Design review of the part built by this model. Coordinates are the model's own, in mm. Face numbers are marked on the shaded views. A direction names the side the tool comes from. Round coordinates to 2 decimals unless told otherwise and drop trailing zeros. Order: outer loops, then holes, each group sorted by start corner. A loop starts at its lowest first (then second) coordinate and runs counter-clockwise, first axis right, second up. Notation, with made-up numbers: M 39,41.25 L 59,41.25 A25 ccw 59,65.25 Z; hole C 11.5,14.5 d5. An arc over 180 degrees is marked long. Write item = value, one per line. Start each with the question number.
```python
from build123d import *

# Parameters (mm, degrees)
SKETCH_1_W          = 15
SKETCH_1_H          = 50
EXTRUDE_1_DEPTH     = 8
SKETCH_2_R          = 1.5
CUT_EXTRUDE_1_DEPTH = 28.299267389
CUT_EXTRUDE_3_DEPTH = 28.299267389


with BuildPart() as part:
    # 草图1 → 凸台-拉伸1 (new body)
    with BuildSketch(Plane.XY):
        Rectangle(SKETCH_1_W, SKETCH_1_H)
    extrude(amount=EXTRUDE_1_DEPTH)

    # 草图2 → 切除-拉伸1 (cut, through all)
    with BuildSketch(Plane.XY.offset(8)):
        with Locations((-4, 21)):
            Circle(SKETCH_2_R)
        with Locations((4, 21)):
            Circle(SKETCH_2_R)
        with Locations((4, -21)):
            Circle(SKETCH_2_R)
        with Locations((-4, -21)):
            Circle(SKETCH_2_R)
    extrude(amount=-CUT_EXTRUDE_1_DEPTH, mode=Mode.SUBTRACT)

    # 草图3 → 切除-拉伸3 (cut, through all)
    with BuildSketch(Plane.XY.offset(8)):
        with BuildLine():
            Line((3.5, 15), (3.5, -15))
            ThreePointArc((3.5, -15), (0, -18.5), (-3.5, -15))
            Line((-3.5, -15), (-3.5, 15))
            ThreePointArc((-3.5, 15), (0, 18.5), (3.5, 15))
        make_face()
    extrude(amount=-CUT_EXTRUDE_3_DEPTH, mode=Mode.SUBTRACT)


solid = part.part
```
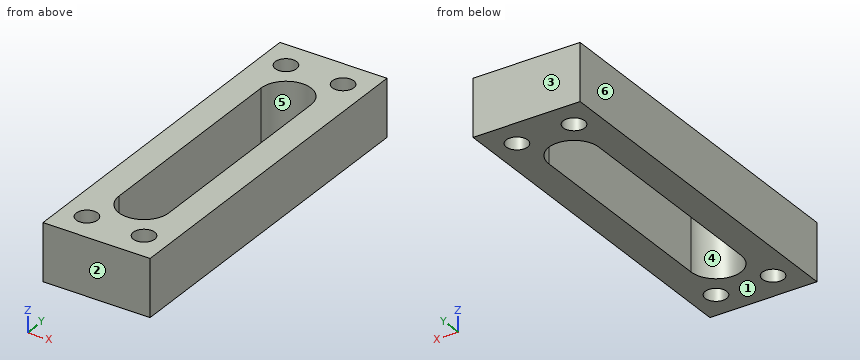
(1) For the marked faces 5 and 6, list the 3-axis set-ups (+Z, -Z, +X, -X, +Y, -Y) from which the entire face can be reached by the end or side of a thin tool; tool diameter is ignored.
(2) Consider section D-D, the plane y = 6. Write out the cut boundary in (x, z), then the cut area to 3 significant figures.
(3) For line 1 along Y through (x, z) = (4, 3); line 2 along X through (y, z) = (7, 3.75); line 3 along Y through (x, z) = (-3, 6.25), list the stretches that pass through material, from the lowest coordinate up. Write a range as [from, to].
(4) Insertion check: pin 1 (6 mm diameter, centred on x = 2, y = 13, fed in from -Z). The pin has a flat end and moves straight along its axis. Give the tip position at first contact, or say it passes through.
(5) Consider section A-A, the plane z = 4.25. Write out the cut boundary in (x, y), then the cut area to 3 significant figures.
(6) Consider section B-B, the plane y = 21. Write out the cut boundary in (x, z).
(7) Consider section C-C, the plane x = 0. Write out the cut boundary in (y, z), then the cut area to 3 significant figures.
(8) Draft analysis for pull direction Y (two halves, no side actions). For the marked faces 1, 2, 3 and 4, state which applies: pulls with the +Y half, pulls with the -Y half, needs draft (parallel to the pull), parting line crosses it, or undercut.
Completed:
q1.face_5 = +Z, -Z
q1.face_6 = +Z, -Z, -X, +Y, -Y
q2.outline = M -7.5,0 L -3.5,0 L -3.5,8 L -7.5,8 Z; M 3.5,0 L 7.5,0 L 7.5,8 L 3.5,8 Z
q2.area = 64.0 mm2
q3.line_1 = [-25, -22.5], [-19.5, 19.5], [22.5, 25]
q3.line_2 = [-7.5, -3.5], [3.5, 7.5]
q3.line_3 = [-25, -22.12], [-19.88, -16.8], [16.8, 19.88], [22.12, 25]
q4.pin_1 = 0
q5.outline = M -7.5,-25 L 7.5,-25 L 7.5,25 L -7.5,25 Z; hole C -4,-21 d3; hole C -4,21 d3; hole M -3.5,-15 A3.5 ccw 3.5,-15 L 3.5,15 A3.5 ccw -3.5,15 Z; hole C 4,-21 d3; hole C 4,21 d3
q5.area = 473 mm2
q6.outline = M -7.5,0 L -5.5,0 L -5.5,8 L -7.5,8 Z; M -2.5,0 L 2.5,0 L 2.5,8 L -2.5,8 Z; M 5.5,0 L 7.5,0 L 7.5,8 L 5.5,8 Z
q7.outline = M -25,0 L -18.5,0 L -18.5,8 L -25,8 Z; M 18.5,0 L 25,0 L 25,8 L 18.5,8 Z
q7.area = 104 mm2
q8.face_1 = needs draft
q8.face_2 = pulls with the -Y half
q8.face_3 = pulls with the +Y half
q8.face_4 = undercut
